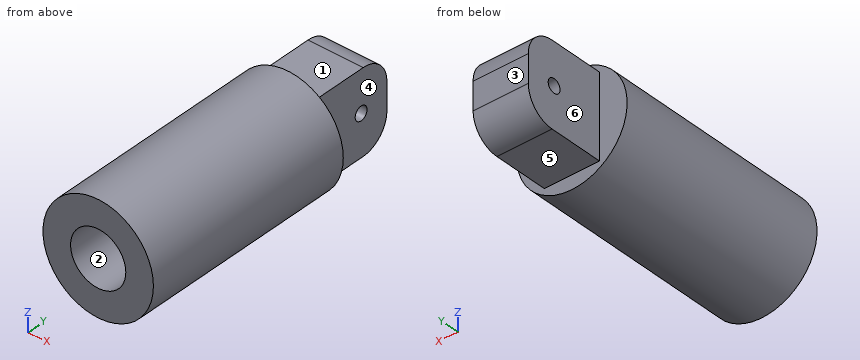
from build123d import *

# Parameters (mm, degrees)
F0_R     = 25.4
F1_DEPTH = 101.6
F2_R     = 12.7
F3_DEPTH = 76.2
F4_W     = 38.1
F4_H     = 38.1
F4_R     = 3.175
F5_DEPTH = 12.7
F6_R     = 12.7


with BuildPart() as f1:
    # F0 (on Front) → F1 (new body)
    with BuildSketch(Plane.XZ):
        Circle(F0_R)
    extrude(amount=F1_DEPTH)

    # F2 (on face) → F3 (cut)
    with BuildSketch(Plane.XZ.offset(101.6)):
        Circle(F2_R)
    extrude(amount=-F3_DEPTH, mode=Mode.SUBTRACT)

    # F4 (on Right) → F5 (join, symmetric)
    with BuildSketch(Plane.YZ):
        with Locations((19.05, 0)):
            Rectangle(F4_W, F4_H)
        with Locations((24.3041142821, 0)):
            Circle(F4_R, mode=Mode.SUBTRACT)
    extrude(amount=F5_DEPTH, both=True)

    # F6
    f6_edges = [f1.edges().sort_by_distance(p)[0] for p in [
        (0, 38.1, 19.05),
        (0, 38.1, -19.05),
    ]]
    fillet(f6_edges, radius=F6_R)


solid = f1.part
Source: CAD feature listing. Evaluate the final solid. Frame: model axes, mm. Face numbers are marked on the shaded views. A direction names the side the tool comes from. Give positions to 0.01 mm unless a question says otherwise; leave off trailing zeros. Write each loop counter-clockwise with the first axis right and the second up, starting at its lowest first coordinate (ties: lowest second). Pieces come first, ordered by that corner, then holes. Notation, with made-up numbers: (-0.5, 41.5) - (6.5, 41.5) arc R28 cw to (6.5, 59.5) - close; hole circle Ø10 at (22.25, 48). An arc over 180 degrees is marked (long way). Write item = value, one per line. Start each with the question number.
Q1. Draft query along Z for the marked faces 1, 2 and 3. Return one class per face: +Z half, -Z half, draft (parallel to the pull), parting line (faces both ways), or undercut.
Q2. Cut plane C-C, the plane z = 9. Return loops of the section in (x, y).
Q3. Pin query (flat end, axial travel): pin 1 Ø4 at (x, y) = (-2.5, -76) entering from +Z; pin 2 Ø10 at (y, z) = (24.3, 0) entering from +X; pin 3 Ø1.5 at (y, z) = (-78, -13) entering from +X. Return the tip coordinate at first contact, or that it passes through.
Q4. Cut plane D-D, the plane x = -8. Return loops of the section in (y, z) (3 decimals), then the cut area to 3 significant figures.
Q5. Material intervals for probe 1 along Z at (x, y) = (0, -62); probe 2 along Z at (x, y) = (-9, 14.5); probe 3 along Y at (x, z) = (2.5, -4.5), sorted ascending.
Q6. Cut plane A-A, the plane z = 0. Return loops of the section in (x, y).
Q7. Cut plane B-B, the plane x = 0. Return loops of the section in (y, z) (3 decimals).
Q8. Reachability of the marked faces 4, 5 and 6 from +Z, -Z, +X, -X, +Y, -Y: full face, straight path, thin tool, end or side. Return the list, or none.
Computed values:
q1.face_1 = +Z half
q1.face_2 = undercut
q1.face_3 = draft
q2.outline = (-23.75, -101.6) - (-8.96, -101.6) - (-8.96, -25.4) - (8.96, -25.4) - (8.96, -101.6) - (23.75, -101.6) - (23.75, 0) - (12.7, 0) - (12.7, 37.82) - (-12.7, 37.82) - (-12.7, 0) - (-23.75, 0) - close
q3.pin_1 = 25.4
q3.pin_2 = 12.7
q3.pin_3 = 22.25
q4.outline = (-101.6, -24.107) - (0, -24.107) - (0, -19.05) - (25.4, -19.05) arc R12.7 ccw to (38.1, -6.35) - (38.1, 6.35) arc R12.7 ccw to (25.4, 19.05) - (0, 19.05) - (0, 24.107) - (-101.6, 24.107) - (-101.6, 9.864) - (-25.4, 9.864) - (-25.4, -9.864) - (-101.6, -9.864) - close; hole circle Ø6.35 at (24.304, 0)
q4.area = 4,750 mm²
q5.probe_1 = -25.4 to -12.7, 12.7 to 25.4
q5.probe_2 = -19.05 to 19.05
q5.probe_3 = -25.4 to 38.1
q6.outline = (-25.4, -101.6) - (-12.7, -101.6) - (-12.7, -25.4) - (12.7, -25.4) - (12.7, -101.6) - (25.4, -101.6) - (25.4, 0) - (12.7, 0) - (12.7, 21.13) - (-12.7, 21.13) - (-12.7, 0) - (-25.4, 0) - close; (-12.7, 27.48) - (12.7, 27.48) - (12.7, 38.1) - (-12.7, 38.1) - close
q7.outline = (-101.6, -25.4) - (0, -25.4) - (0, -19.05) - (25.4, -19.05) arc R12.7 ccw to (38.1, -6.35) - (38.1, 6.35) arc R12.7 ccw to (25.4, 19.05) - (0, 19.05) - (0, 25.4) - (-101.6, 25.4) - (-101.6, 12.7) - (-25.4, 12.7) - (-25.4, -12.7) - (-101.6, -12.7) - close; hole circle Ø6.35 at (24.304, 0)
q8.face_4 = +Z, -Z, +X, +Y
q8.face_5 = -Z, +X, -X, +Y
q8.face_6 = +Z, -Z, -X, +Y
